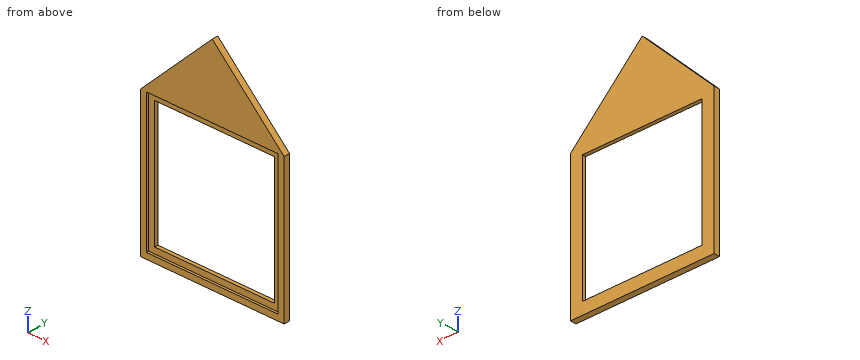
```python
from build123d import *

# Parameters (mm, degrees)
F0_W     = 152.4
F0_H     = 152.4
F1_DEPTH = 6.35
F2_W     = 139.7
F2_H     = 146.05
F3_DEPTH = 2.54
F4_W     = 127
F4_H     = 133.35
F5_DEPTH = 3.811


with BuildPart() as f1:
    # F0 (on Front) → F1 (new body)
    with BuildSketch(Plane.XZ):
        Polygon((76.2, 76.2), (0, 0), (152.4, 0), align=None)
        with Locations((76.2, -76.2)):
            Rectangle(F0_W, F0_H)
    extrude(amount=F1_DEPTH)

    # F2 (on face) → F3 (cut)
    with BuildSketch(Plane.XZ.offset(6.35)):
        with Locations((76.2, -73.025)):
            Rectangle(F2_W, F2_H)
    extrude(amount=-F3_DEPTH, mode=Mode.SUBTRACT)

    # F4 (on face) → F5 (cut, through all)
    with BuildSketch(Plane.XZ.offset(3.81)):
        with Locations((76.2, -73.025)):
            Rectangle(F4_W, F4_H)
    extrude(amount=-F5_DEPTH, mode=Mode.SUBTRACT)


solid = f1.part
```
Read the model definition and answer for the solid it produces. Units are mm, in the model's axes. Give positions to 0.01 mm unless a question says otherwise; leave off trailing zeros. Loops run counter-clockwise (first coordinate to the right, second up) from the corner with the lowest first, then second, coordinate; pieces in that order, holes last.
Item 1: The part is cut by section A-A (x = 44). Write down the section's boundary in (y, z).
Item 2: Find the intervals of material crossed by line 1 along X through (y, z) = (-3.75, -115); line 2 along X through (y, z) = (-4.25, -20); line 3 along Z through (x, y) = (83, -5), in increasing order.
Item 3: Each of these flat-tipped pins is pushed along its axis until it touches: pin 1 Ø1.3 at (x, y) = (91, -5) entering from +Z; pin 2 Ø1.1 at (y, z) = (-2.5, -70) entering from -X; pin 3 Ø1.1 at (x, y) = (72.5, -2.5) entering from +Z. Where does it stop, or does it pass through?
Item 4: The part is cut by section D-D (z = 26). Write down the section's boundary in (x, y).
Item 5: The part is cut by section B-B (z = -110.5). Write down the section's boundary in (x, y), and give its area (3 significant figures).
Item 6: The part is cut by section C-C (y = -1.5). Write down the section's boundary in (x, z), and give its area (3 significant figures).
Taken from the geometry:
1. outline: (-6.35, -152.4) - (0, -152.4) - (0, -139.7) - (-3.81, -139.7) - (-3.81, -146.05) - (-6.35, -146.05) - close; (-6.35, 0) - (-3.81, 0) - (-3.81, -6.35) - (0, -6.35) - (0, 44) - (-6.35, 44) - close
2. line 1: x = 0 to 12.7, 139.7 to 152.4
2. line 2: x = 0 to 6.35, 146.05 to 152.4
2. line 3: z = -152.4 to -146.05, 0 to 69.4
3. pin 1: stops at z = 62.05
3. pin 2: stops at x = 0
3. pin 3: stops at z = 73.05
4. outline: (26, -6.35) - (126.4, -6.35) - (126.4, 0) - (26, 0) - close
5. outline: (0, -6.35) - (6.35, -6.35) - (6.35, -3.81) - (12.7, -3.81) - (12.7, 0) - (0, 0) - close; (139.7, -3.81) - (146.05, -3.81) - (146.05, -6.35) - (152.4, -6.35) - (152.4, 0) - (139.7, 0) - close
5. area: 129 mm2
6. outline: (0, -152.4) - (152.4, -152.4) - (152.4, 0) - (76.2, 76.2) - (0, 0) - close; hole (12.7, -139.7) - (139.7, -139.7) - (139.7, -6.35) - (12.7, -6.35) - close
6. area: 12,100 mm2
